Autodesk Inventor part; units mm, degrees
ref_plane "YZ Plane" through (0, 0, 0) normal (1, 0, 0) x (0, 1, 0)
ref_plane "XZ Plane" through (0, 0, 0) normal (0, 1, 0) x (-1, 0, 0)
ref_plane "XY Plane" through (0, 0, 0) normal (0, 0, 1) x (1, 0, 0)
sketch "Sketch1" plane through (0, 0, 0) normal (1, 0, 0) x (0, 1, 0)
  line L0 (10.7385, 7.5) -> (-10.7385, 7.5)
  line L1 (-10.7385, 7.5) -> (-10.7385, -7.5)
  line L2 (-10.7385, -7.5) -> (10.7385, -7.5)
  line L3 (10.7385, -7.5) -> (10.7385, 7.5)
  point P0 (0, 0)
  dimension "d0" = 21.477
  dimension "d1" = 15
  dimension "d2" = 10.7385
  dimension "d3" = 7.5
extrude "Extrusion1" add sketch "Sketch1" along normal blind 9
sketch "Sketch2" plane through (9, 0, 0) normal (1, 0, 0) x (0, 0, -1)
  line L0 (7.5, 10.7385) -> (-7.5, 10.7385)
  arc A0 (-1.5, 10.7385) -> (1.5, 10.7385) centre (0, 10.7385) ccw
  point P0 (0, 0)
  dimension "d8" = 3
extrude "Extrusion2" cut sketch "Sketch2" against normal through all
sketch "Sketch3" plane through (9, 0, 0) normal (1, 0, 0) x (0, 0, -1)
  circle A0 centre (3.983, 6.2605) radius 1.5
  arc A1 (-1.5, 10.7385) -> (1.5, 10.7385) centre (0, 10.7385) ccw
  line L0 (7.5, 10.7385) -> (1.5, 10.7385)
  point P0 (0, 0)
  dimension "d12" = 3
  dimension "d13" = 3.983
  dimension "d14" = 4.478
extrude "Extrusion3" add sketch "Sketch3" along normal blind 3
sketch "Sketch4" plane through (0, 0, 0) normal (-1, 0, 0) x (0, 0, 1)
  line L0 (-2.5186, -3.6831) -> (10.3419, -3.6831) construction
  line L1 (10.3419, -3.6831) -> (10.3419, -8.8157) construction
  line L2 (10.3419, -8.8157) -> (-2.5186, -8.8157) construction
  line L3 (-2.5186, -8.8157) -> (-2.5186, -3.6831) construction
  line L4 (-0.5697, -6.741) -> (-2.0567, -6.741)
  line L5 (-2.0567, -6.741) -> (-2.0567, -6.4297)
  line L6 (-2.0567, -6.4297) -> (-1.5034, -6.4297)
  line L7 (-1.5034, -6.4297) -> (-1.5034, -4.387)
  line L8 (-1.5034, -4.387) -> (-2.0567, -4.387)
  line L9 (-2.0567, -4.387) -> (-2.0567, -4.1079)
  spline S0 degree 2 poles (-2.0567, -4.1079) (-1.743, -4.1079) (-1.4466, -3.9301) (-1.4268, -3.6831) knots 0 0 0 1 2 2 2
  line L10 (-1.4268, -3.6831) -> (-1.1106, -3.6831)
  line L11 (-1.1106, -3.6831) -> (-1.1106, -6.4297)
  line L12 (-1.1106, -6.4297) -> (-0.5697, -6.4297)
  line L13 (-0.5697, -6.4297) -> (-0.5697, -6.741)
  line L14 (-0.2511, -6.741) -> (0.7764, -3.693)
  line L15 (0.7764, -3.693) -> (1.2754, -3.693)
  line L16 (1.2754, -3.693) -> (2.3029, -6.741)
  line L17 (2.3029, -6.741) -> (1.8756, -6.741)
  line L18 (1.8756, -6.741) -> (1.599, -5.8888)
  line L19 (1.599, -5.8888) -> (0.4356, -5.8888)
  line L20 (0.4356, -5.8888) -> (0.1589, -6.741)
  line L21 (0.1589, -6.741) -> (-0.2511, -6.741)
  line L22 (1.4878, -5.543) -> (1.016, -4.1079)
  line L23 (1.016, -4.1079) -> (0.5467, -5.543)
  line L24 (0.5467, -5.543) -> (1.4878, -5.543)
  point P0 (0, 0)
emboss "Emboss1" sketch "Sketch4" operation cut depth 1 direction (1, 0, 0)
properties part number "Support_1A"
Read the model definition and answer for the solid it produces. Units are mm, in the model's axes. A direction names the side the tool comes from. Coordinates: 2 decimals unless noted, no trailing zeros. Loops run counter-clockwise (first coordinate to the right, second up) from the corner with the lowest first, then second, coordinate; pieces in that order, holes last. Notation, with made-up numbers: (30, -12.75) - (56, -12.75) arc R13 cw to (56, -3.75) - close; hole circle Ø5 at (56, -1.5). An arc over 180 degrees is marked (long way). Answer in a Markdown table with one row per item.
1. Find section B-B, the plane z = -5.75. Write down the section's boundary in (x, y), then the cut area to 3 significant figures.
Conclusion:
| item | result |
|---|---|
| outline | (0, -10.74) - (9, -10.74) - (9, 10.74) - (0, 10.74) - close |
| area | 193 mm² |
2. Determine the mould class of faces 3 (the face through (12, 6, -4)), 4 (the face through (1, -5.2, -1.3)), 5 (the face through (4, 10.738, -5)) for opening direction Y: +Y half, -Y half, draft (parallel to the pull), parting line (faces both ways), or undercut.
Conclusion:
| item | result |
|---|---|
| face 3 | draft |
| face 4 | undercut |
| face 5 | +Y half |
3. Find section C-C, the plane x = 10.5. Write down the section's boundary in (y, z).
Conclusion:
| item | result |
|---|---|
| outline | circle Ø3 at (6.26, -3.98) |
4. Find section A-A, the plane y = 5.75. Write down the section's boundary in (x, z), then the cut area to 3 significant figures.
Conclusion:
| item | result |
|---|---|
| outline | (0, -7.5) - (9, -7.5) - (9, -5.39) - (12, -5.39) - (12, -2.57) - (9, -2.57) - (9, 7.5) - (0, 7.5) - close |
| area | 143 mm² |
5. Straight lines are drawn through the part: line 1 (X direction, y = 6.5, z = -1.75); line 2 (Y direction, x = 2.75, z = 0.25); line 3 (Y direction, x = 2.75, z = -1). For each, find the intervals that lie inside material, in ascending order.
Conclusion:
| item | result |
|---|---|
| line 1 | x = 0 to 9 |
| line 2 | y = -10.74 to 9.26 |
| line 3 | y = -10.74 to 9.62 |
6. Which of the six approach directions +Z, -Z, +X, -X, +Y, -Y give full straight-line access (tool end or side, diameter ignored) to faces 1 (the face through (4, 10.738, 4)), 2 (the face through (0.493, -5.238, 0.255))?
Conclusion:
| item | result |
|---|---|
| face 1 | +Z, -Z, +X, -X, +Y |
| face 2 | -X |
7. Find section D-D, the plane y = -9.5. Write down the section's boundary in (x, z), then the cut area to 3 significant figures.
Conclusion:
| item | result |
|---|---|
| outline | (0, -7.5) - (9, -7.5) - (9, 7.5) - (0, 7.5) - close |
| area | 135 mm² |
8. Given pin 1 (7.5 mm diameter, centred on y = -1, z = -1, fed in from +X), flat-ended and moving along its own axis, determine where the tip first touches the part or whether it passes through.
Conclusion:
| item | result |
|---|---|
| pin 1 | stops at x = 9 |
